Source: CAD feature listing. Evaluate the final solid. Frame: model axes, mm. Face numbers are marked on the shaded views. Give positions to 0.01 mm unless a question says otherwise; leave off trailing zeros. Write each loop counter-clockwise with the first axis right and the second up, starting at its lowest first coordinate (ties: lowest second). Pieces come first, ordered by that corner, then holes. Notation, with made-up numbers: M 53.5,25 L 79.5,25 A21 ccw 79.5,44 Z; hole C 69,-19.75 d4. An arc over 180 degrees is marked long. Return JSON: item names as keys, results as strings.
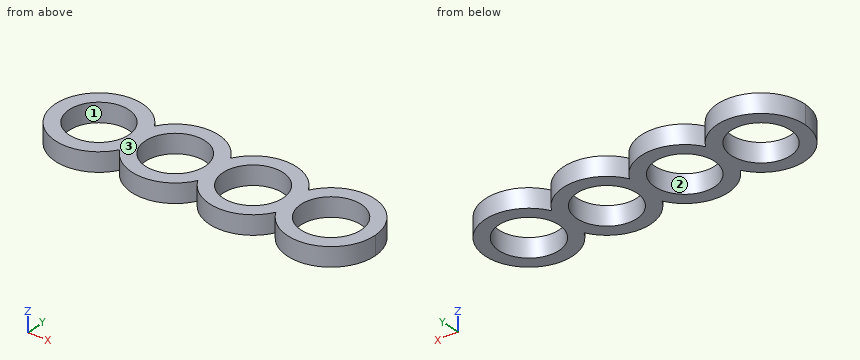
```python
from build123d import *

# Parameters (mm, degrees)
F1_DEPTH = 7


with BuildPart() as f1:
    # F0 (on Top) → F1 (new body)
    with BuildSketch(Plane.XY):
        with BuildLine():
            Line((-31.3795059258, 0), (-26.922398242, 0))
            ThreePointArc((-26.922398242, 0), (-27.4894668745, 4.2460498939), (-29.1509244493, 8.1944755629))
            ThreePointArc((-29.1509244493, 8.1944755629), (-30.8124227539, 4.246057146), (-31.3795059258, 0))
        make_face()
        with BuildLine():
            Line((-26.2997059258, 0), (-26.922398242, 0))
            ThreePointArc((-26.922398242, 0), (-27.4894668745, -4.2460498939), (-29.1509244493, -8.1944755629))
            ThreePointArc((-29.1509244493, -8.1944755629), (-14.9190087878, -16.1773649633), (-0.9726024938, -7.7055470911))
            ThreePointArc((-0.9726024938, -7.7055470911), (-2.4295294135, -3.9745590906), (-2.9252990617, 0))
            Line((-2.9252990617, 0), (-4.0997059258, 0))
            ThreePointArc((-4.0997059258, 0), (-15.1997059258, -11.1), (-26.2997059258, 0))
        make_face()
        with BuildLine():
            ThreePointArc((-29.1509244493, 8.1944755629), (-27.4894668745, 4.2460498939), (-26.922398242, 0))
            Line((-26.922398242, 0), (-26.2997059258, 0))
            ThreePointArc((-26.2997059258, 0), (-15.1997059258, 11.1), (-4.0997059258, 0))
            Line((-4.0997059258, 0), (-2.9252990617, 0))
            ThreePointArc((-2.9252990617, 0), (-2.4295294135, 3.9745590906), (-0.9726024938, 7.7055470911))
            ThreePointArc((-0.9726024938, 7.7055470911), (-14.9190087878, 16.1773649633), (-29.1509244493, 8.1944755629))
        make_face()
        with BuildLine():
            ThreePointArc((-29.1509244493, -8.1944755629), (-27.4894668745, -4.2460498939), (-26.922398242, 0))
            Line((-26.922398242, 0), (-31.3795059258, 0))
            ThreePointArc((-31.3795059258, 0), (-30.8124227539, -4.246057146), (-29.1509244493, -8.1944755629))
        make_face()
        with BuildLine():
            ThreePointArc((-31.3795059258, 0), (-30.8124227539, 4.246057146), (-29.1509244493, 8.1944755629))
            ThreePointArc((-29.1509244493, 8.1944755629), (-47.3485941376, 15.6130773691), (-59.2826902453, 0))
            Line((-59.2826902453, 0), (-54.1525442436, 0))
            ThreePointArc((-54.1525442436, 0), (-43.1025442436, 11.05), (-32.0525442436, 0))
            Line((-32.0525442436, 0), (-31.3795059258, 0))
        make_face()
        with BuildLine():
            ThreePointArc((-59.2826902453, 0), (-47.3485941376, -15.6130773691), (-29.1509244493, -8.1944755629))
            ThreePointArc((-29.1509244493, -8.1944755629), (-30.8124227539, -4.246057146), (-31.3795059258, 0))
            Line((-31.3795059258, 0), (-32.0525442436, 0))
            ThreePointArc((-32.0525442436, 0), (-43.1025442436, -11.05), (-54.1525442436, 0))
            Line((-54.1525442436, 0), (-59.2826902453, 0))
        make_face()
        with BuildLine():
            ThreePointArc((27.5160949741, 7.6415223351), (13.2908629072, 16.1797591406), (-0.9726024938, 7.7055470911))
            ThreePointArc((-0.9726024938, 7.7055470911), (0.4843244259, 3.9745590906), (0.9800940742, 0))
            Line((0.9800940742, 0), (2.1045009383, 0))
            ThreePointArc((2.1045009383, 0), (13.2545009383, 11.15), (24.4045009383, 0))
            Line((24.4045009383, 0), (25.5978890099, 0))
            ThreePointArc((25.5978890099, 0), (26.0847659676, 3.9393012616), (27.5160949741, 7.6415223351))
        make_face()
        with BuildLine():
            ThreePointArc((0.9800940742, 0), (0.4843244259, 3.9745590906), (-0.9726024938, 7.7055470911))
            ThreePointArc((-0.9726024938, 7.7055470911), (-2.4295294135, 3.9745590906), (-2.9252990617, 0))
            Line((-2.9252990617, 0), (0, 0))
            Line((0, 0), (0.9800940742, 0))
        make_face()
        with BuildLine():
            ThreePointArc((-2.9252990617, 0), (-2.4295294135, -3.9745590906), (-0.9726024938, -7.7055470911))
            ThreePointArc((-0.9726024938, -7.7055470911), (0.4843244259, -3.9745590906), (0.9800940742, 0))
            Line((0.9800940742, 0), (0, 0))
            Line((0, 0), (-2.9252990617, 0))
        make_face()
        with BuildLine():
            ThreePointArc((0.9800940742, 0), (0.4843244259, -3.9745590906), (-0.9726024938, -7.7055470911))
            ThreePointArc((-0.9726024938, -7.7055470911), (13.2908629072, -16.1797591406), (27.5160949741, -7.6415223351))
            ThreePointArc((27.5160949741, -7.6415223351), (26.0847659676, -3.9393012616), (25.5978890099, 0))
            Line((25.5978890099, 0), (24.4045009383, 0))
            ThreePointArc((24.4045009383, 0), (13.2545009383, -11.15), (2.1045009383, 0))
            Line((2.1045009383, 0), (0.9800940742, 0))
        make_face()
        with BuildLine():
            ThreePointArc((57.9574890099, 0), (45.7169902715, 15.6929230423), (27.5160949741, 7.6415223351))
            ThreePointArc((27.5160949741, 7.6415223351), (28.9474239806, 3.9393012616), (29.4343009383, 0))
            Line((29.4343009383, 0), (30.5776890099, 0))
            ThreePointArc((30.5776890099, 0), (41.7776890099, 11.2), (52.9776890099, 0))
            Line((52.9776890099, 0), (57.9574890099, 0))
        make_face()
        with BuildLine():
            ThreePointArc((29.4343009383, 0), (28.9474239806, 3.9393012616), (27.5160949741, 7.6415223351))
            ThreePointArc((27.5160949741, 7.6415223351), (26.0847659676, 3.9393012616), (25.5978890099, 0))
            Line((25.5978890099, 0), (29.4343009383, 0))
        make_face()
        with BuildLine():
            ThreePointArc((25.5978890099, 0), (26.0847659676, -3.9393012616), (27.5160949741, -7.6415223351))
            ThreePointArc((27.5160949741, -7.6415223351), (28.9474239806, -3.9393012616), (29.4343009383, 0))
            Line((29.4343009383, 0), (25.5978890099, 0))
        make_face()
        with BuildLine():
            ThreePointArc((29.4343009383, 0), (28.9474239806, -3.9393012616), (27.5160949741, -7.6415223351))
            ThreePointArc((27.5160949741, -7.6415223351), (45.7169902715, -15.6929230423), (57.9574890099, 0))
            Line((57.9574890099, 0), (52.9776890099, 0))
            ThreePointArc((52.9776890099, 0), (41.7776890099, -11.2), (30.5776890099, 0))
            Line((30.5776890099, 0), (29.4343009383, 0))
        make_face()
    extrude(amount=F1_DEPTH)


solid = f1.part
```
1) Line query: line 1 (X direction, y = -2.5, z = 4.75); line 2 (X direction, y = 0.5, z = 1); line 3 (X direction, y = -14, z = 0.5). Output: solid intervals per line, ascending. Write a range as [from, to].
Numbers:
{"line 1": "x = [-59.09, -53.87], [-32.34, -26.01], [-4.38, 2.39], [24.12, 30.86], [52.7, 57.76]", "line 2": "x = [-59.27, -54.14], [-32.06, -26.29], [-4.11, 2.12], [24.39, 30.59], [52.97, 57.95]", "line 3": "x = [-51.21, -34.99], [-23.31, -7.09], [5.14, 21.37], [33.67, 49.89]"}
2) Cut plane C-C, the plane z = 1.75. Return the cut outline in (x, y).
Numbers:
{"outline": "M -29.15,-8.19 A16.18 ccw -0.97,-7.71 A16.18 ccw 27.52,-7.64 A16.18 ccw long 27.52,7.64 A16.18 ccw -0.97,7.71 A16.18 ccw -29.15,8.19 A16.18 ccw long Z; hole C -43.1,0 d22.1; hole C -15.2,0 d22.2; hole C 13.25,0 d22.3; hole C 41.78,0 d22.4"}
3) Cut plane A-A, the plane y = -1.5. Return the cut outline in (x, z).
Numbers:
{"outline": "M -59.21,0 L -54.05,0 L -54.05,7 L -59.21,7 Z; M -32.15,0 L -26.2,0 L -26.2,7 L -32.15,7 Z; M -4.2,0 L 2.21,0 L 2.21,7 L -4.2,7 Z; M 24.3,0 L 30.68,0 L 30.68,7 L 24.3,7 Z; M 52.88,0 L 57.89,0 L 57.89,7 L 52.88,7 Z"}
4) Cut plane B-B, the plane x = -43.5. Return the cut outline in (y, z).
Numbers:
{"outline": "M -16.18,0 L -11.04,0 L -11.04,7 L -16.18,7 Z; M 11.04,0 L 16.18,0 L 16.18,7 L 11.04,7 Z"}
5) Draft query along X for the marked faces 1, 2 and 3. Return one class per face: released by +X, released by -X, zero draft, split by the parting line, or undercut.
Numbers:
{"face 1": "undercut", "face 2": "undercut", "face 3": "zero draft"}
6) Cut plane D-D, the plane x = -19. Return the cut outline in (y, z).
Numbers:
{"outline": "M -15.73,0 L -10.43,0 L -10.43,7 L -15.73,7 Z; M 10.43,0 L 15.73,0 L 15.73,7 L 10.43,7 Z"}
7) Contact query for flat-ended pins moving along their axis: pin 1 Ø4 at (x, z) = (-29.5, 2.5) entering from -Y; pin 2 Ø3 at (x, z) = (35.5, 3) entering from +Y; pin 3 Ø1.5 at (x, z) = (-19.5, 5.5) entering from +Y. Output: stop coordinate, or through.
Numbers:
{"pin 1": "stops at y = -11.28", "pin 2": "stops at y = 15.46", "pin 3": "stops at y = 15.79"}
